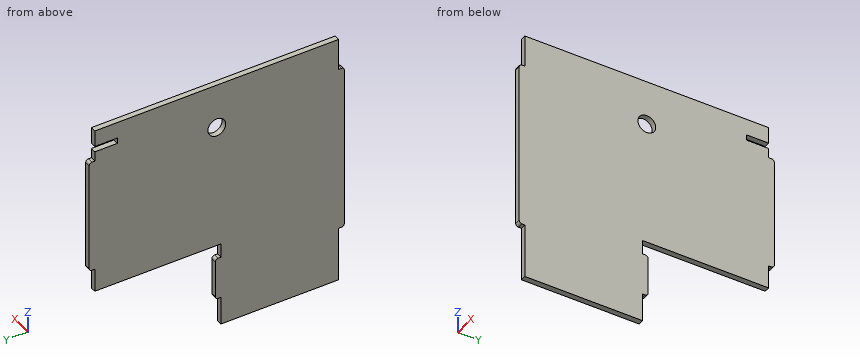
```python
from build123d import *

# Parameters (mm, degrees)
SKETCH2_R           = 3.17
BOSS_EXTRUDE1_DEPTH = 2


with BuildPart() as part:
    # Sketch2 → Boss-Extrude1 (new body)
    with BuildSketch(Plane(origin=(0, 0, 0), x_dir=(0, 0, -1), z_dir=(1, 0, 0))):
        with BuildLine():
            Line((44.752383591, -64.243785516), (44.752383591, -22.243785516))
            Line((44.752383591, -22.243785516), (34.752383591, -22.243785516))
            Line((34.752383591, -22.243785516), (34.752383591, -21.243785516))
            ThreePointArc((34.752383591, -21.243785516), (34.459490372, -20.536678734), (33.752383591, -20.243785516))
            Line((33.752383591, -20.243785516), (20.752383591, -20.243785516))
            ThreePointArc((20.752383591, -20.243785516), (20.045276809, -20.536678734), (19.752383591, -21.243785516))
            Line((19.752383591, -21.243785516), (19.752383591, -22.243785516))
            Line((19.752383591, -22.243785516), (14.752383591, -22.243785516))
            Line((14.752383591, -22.243785516), (14.752383591, 22.756214484))
            Line((14.752383591, 22.756214484), (6.501874719, 22.756214484))
            Line((6.501874719, 22.756214484), (6.501874719, 23.756214484))
            ThreePointArc((6.501874719, 23.756214484), (6.2089815, 24.463321266), (5.501874719, 24.756214484))
            Line((5.501874719, 24.756214484), (-32.997107538, 24.756214484))
            ThreePointArc((-32.997107538, 24.756214484), (-33.704214319, 24.463321266), (-33.997107538, 23.756214484))
            Line((-33.997107538, 23.756214484), (-33.997107538, 22.756214484))
            Line((-33.997107538, 22.756214484), (-37.447616409, 22.756214484))
            Line((-37.447616409, 22.756214484), (-37.447616409, 14.756214484))
            Line((-37.447616409, 14.756214484), (-39.447616409, 14.756214484))
            Line((-39.447616409, 14.756214484), (-39.447616409, 22.756214484))
            Line((-39.447616409, 22.756214484), (-45.247616409, 22.756214484))
            Line((-45.247616409, 22.756214484), (-45.247616409, -64.243785516))
            Line((-45.247616409, -64.243785516), (-33.997107538, -64.243785516))
            Line((-33.997107538, -64.243785516), (-33.997107538, -65.243785516))
            ThreePointArc((-33.997107538, -65.243785516), (-33.704214319, -65.950892297), (-32.997107538, -66.243785516))
            Line((-32.997107538, -66.243785516), (24.501874719, -66.243785516))
            ThreePointArc((24.501874719, -66.243785516), (25.2089815, -65.950892297), (25.501874719, -65.243785516))
            Line((25.501874719, -65.243785516), (25.501874719, -64.243785516))
            Line((25.501874719, -64.243785516), (44.752383591, -64.243785516))
        make_face()
        with Locations((-29.447616409, -20.743785516)):
            Circle(SKETCH2_R, mode=Mode.SUBTRACT)
    extrude(amount=BOSS_EXTRUDE1_DEPTH)


solid = part.part
```
Geometry check sheet. Reference: the model listing, model coordinates, mm. Coordinates: 2 decimals unless noted, no trailing zeros. Loops run counter-clockwise (first coordinate to the right, second up) from the corner with the lowest first, then second, coordinate; pieces in that order, holes last. Notation, with made-up numbers: (-19, 66.5) - (16, 66.5) arc R31 ccw to (16, 102.5) - close; hole circle Ø3 at (19.25, -3). An arc over 180 degrees is marked (long way). One line per item, written item: value. Start each with the question number.
(1) Depth check by flat-ended pin: P1, Ø0.6, axis at x = 1, z = 38.5, coming from the +Y side; P2, Ø0.6, axis at x = 0.5, y = 17.5, coming from the -Z side; P3, Ø0.5, axis at x = 1, y = -65, coming from the +Z side; P4, Ø5, axis at y = -20.74, z = 29.45, coming from the +X side. Enter the tip coordinate at first touch or a pass-through.
(2) Cross-section at C-C on y = -13. Enter the section's corners in (x, z).
(3) Cross-section at D-D on z = -16. Enter the section's corners in (x, y).
(4) Cross-section at A-A on z = 31. Enter the section's corners in (x, y), plus the area to 3 significant figures.
(5) Material ranges on line 1 (Z direction, x = 1.3, y = 17.5); line 2 (Y direction, x = 1.45, z = -13.5); line 3 (Z direction, x = 1.4, y = -12), recorded low to high. Write a range as [from, to].
Results below:
1. P1: stops at y = 14.76
1. P2: stops at z = -14.75
1. P3: stops at z = 34
1. P4: passes through
2. outline: (0, -14.75) - (2, -14.75) - (2, 45.25) - (0, 45.25) - close
3. outline: (0, -66.24) - (2, -66.24) - (2, -22.24) - (0, -22.24) - close
4. outline: (0, -66.24) - (2, -66.24) - (2, -23.51) - (0, -23.51) - close; (0, -17.98) - (2, -17.98) - (2, 24.76) - (0, 24.76) - close
4. area: 171 mm2
5. line 1: z = [-14.75, 37.45], [39.45, 45.25]
5. line 2: y = [-66.24, 22.76]
5. line 3: z = [-14.75, 45.25]
